For this review, take the finished solid that the model builds, in its own axes (mm). A direction names the side the tool comes from. Coordinates: 2 decimals unless noted, no trailing zeros. Write each loop counter-clockwise with the first axis right and the second up, starting at its lowest first coordinate (ties: lowest second). Pieces come first, ordered by that corner, then holes.
```python
from build123d import *

# Parameters (mm, degrees)
SKETCH_1_R               = 30
EXTRUDE_1_DEPTH          = 3
SKETCH_2_W               = 11
SKETCH_2_H               = 11
EXTRUDE_2_DEPTH          = 4
SKETCH_4_R               = 6
CUT_EXTRUDE_1_DEPTH      = 25
SKETCH_5_R               = 9
CUT_EXTRUDE_2_DEPTH      = 9
CUT_EXTRUDE_START        = 7.85
SKETCH_6_R               = 10
SKETCH_6_R_2             = 9
CUT_EXTRUDE_3_DEPTH      = 1.1
SKETCH_8_R               = 26.5
EXTRUDE_3_DEPTH          = 5
CUT_EXTRUDE_4_DEPTH      = 92.299851037
CUT_EXTRUDE_4_DEPTH_BACK = 92.299851037
SKETCH_7_R               = 15
SKETCH_10_R              = 2.25
CUT_EXTRUDE_5_DEPTH      = 17


with BuildPart() as part:
    # Sketch 1 → Extrude 1 (new body)
    with BuildSketch(Plane.XY):
        Circle(SKETCH_1_R)
    extrude(amount=EXTRUDE_1_DEPTH)



with BuildPart() as body_2:
    # Sketch 2 → Revolve 1 (revolve)
    with BuildSketch(Plane.XY.offset(3)):
        with Locations((68.415621645, -0.125)):
            Rectangle(SKETCH_2_W, SKETCH_2_H)
    revolve(axis=Axis((73.915621645, 22.717290725, 3), (0, -1, 0)))


with BuildPart() as part_1:
    add(part.part)

    add(body_2.part)  # Extrude 2 merges body 2
    # Sketch 3 → Extrude 2 (add, symmetric)
    with BuildSketch(Plane.XY.offset(3)):
        with BuildLine():
            Line((11.214731114, 27.824985284), (66.915621645, 5.375))
            Line((66.915621645, 5.375), (66.915621645, -4))
            Line((66.915621645, -4), (11.80104521, -27.581430926))
            ThreePointArc((11.80104521, -27.581430926), (-29.998320441, -0.317444067), (11.214731114, 27.824985284))
        make_face()
    extrude(amount=EXTRUDE_2_DEPTH, both=True)

    # Sketch 4 → Cut-Extrude 1 (cut)
    with BuildSketch(Plane.XZ.offset(5.625)):
        with Locations(Location((73.915621645, 3, 0), (0, 0, 270))):
            Circle(SKETCH_4_R)
    extrude(amount=-CUT_EXTRUDE_1_DEPTH, mode=Mode.SUBTRACT)

    # Sketch 5 → Cut-Extrude 2 (cut)
    with BuildSketch(Plane.XZ.offset(5.625)):
        with Locations(Location((73.915621645, 3, 0), (0, 0, 270))):
            Circle(SKETCH_5_R)
    extrude(amount=-CUT_EXTRUDE_2_DEPTH, mode=Mode.SUBTRACT)

    # Sketch 6 → Cut-Extrude 3 (cut)
    # profile 1 of 2: a face of its own
    with BuildSketch(Plane.XZ.offset(-3.375).offset(CUT_EXTRUDE_START)):
        with Locations(Location((73.915621645, 3, 0), (0, 0, 270))):
            Circle(SKETCH_6_R)
        with Locations(Location((73.915621645, 3, 0), (0, 0, 270))):
            Circle(SKETCH_6_R_2, mode=Mode.SUBTRACT)
    # profile 2 of 2: a face of its own
    with BuildSketch(Plane.XZ.offset(-3.375).offset(CUT_EXTRUDE_START)):
        with Locations(Location((73.915621645, 3, 0), (0, 0, 270))):
            Circle(SKETCH_6_R_2)
    extrude(amount=-CUT_EXTRUDE_3_DEPTH, mode=Mode.SUBTRACT)

    # Sketch 8 → Extrude 3 (add, symmetric)
    with BuildSketch(Plane(origin=(0, 0, 3), x_dir=(-1, 0, 0), z_dir=(0, 0, -1))):
        with Locations(Location((0, 0, 0), (0, 0, 180))):
            Circle(SKETCH_8_R)
    extrude(amount=EXTRUDE_3_DEPTH, both=True)

    # Sketch 7 → Cut-Extrude 4 (cut, two sides: drawn at the far end of the back side and taken through both)
    with BuildSketch(Plane.XY.offset(7).offset(-CUT_EXTRUDE_4_DEPTH_BACK)):
        with Locations(Location((0, 0, 0), (0, 0, 180))):
            Circle(SKETCH_7_R)
        with BuildLine():
            Line((25.989694724, -14.984517615), (51.662735414, -4))
            Line((51.662735414, -4), (29.732137495, -4))
            ThreePointArc((29.732137495, -4), (28.397104663, -9.674939108), (25.989694724, -14.984517615))
        make_face()
        with BuildLine():
            Line((29.732137495, 4), (51.662735414, 4))
            Line((51.662735414, 4), (25.989694724, 14.984517615))
            ThreePointArc((25.989694724, 14.984517615), (28.397104663, 9.674939108), (29.732137495, 4))
        make_face()
    extrude(amount=CUT_EXTRUDE_4_DEPTH + CUT_EXTRUDE_4_DEPTH_BACK, mode=Mode.SUBTRACT)

    # Sketch 10 → Cut-Extrude 5 (cut)
    with BuildSketch(Plane.XY.offset(8)):
        with Locations((21.75, 0)):
            Circle(SKETCH_10_R)
        with Locations((13.980630511, -16.661466638)):
            Circle(SKETCH_10_R)
        with Locations(Location((-21.75, 0, 0), (0, 0, 180))):
            Circle(SKETCH_10_R)
        with Locations(Location((-13.980630511, -16.661466638, 0), (0, 0, 180))):
            Circle(SKETCH_10_R)
        with Locations(Location((13.980630511, 16.661466638, 0), (0, 0, 180))):
            Circle(SKETCH_10_R)
        with Locations((-13.980630511, 16.661466638)):
            Circle(SKETCH_10_R)
    extrude(amount=-CUT_EXTRUDE_5_DEPTH, mode=Mode.SUBTRACT)


solid = part_1.part
```
1) Consider section D-D (z = 3.25). Count the separate pieces of the cut face and the enclosed holes in it, then the cut area to 3 significant figures.
2) Consider section C-C (x = 28). Give the boundary of the cut face in (y, z), then the cut area to 3 significant figures.
3) Clearance check with flat-ended pins moving along their axes: P1, Ø6.5, axis at x = 77, z = -0.5, coming from the -Y side (3 decimals); P2, Ø10, axis at x = -15, y = 14.5, coming from the +Z side; P3, Ø6.5, axis at x = 43.5, z = 3, coming from the +Y side. State where each tip first meets the part, or that it passes through.
4) For L1, parallel to X at y = -5.3, z = 3; L2, parallel to X at y = -6, z = 4.5; L3, parallel to X at y = -5.05, z = 3, list the stretches that pass through material, from the lowest coordinate up.
5) Consider section B-B (x = 76). Give the boundary of the cut face in (y, z) (3 decimals).
6) Consider section A-A (y = 7). Give the boundary of the cut face in (x, z).
7) The part is to be moulded in two halves that separate along Y. For faces 5 (the face through (-3.45, -26.274, 7.493)), 6 (the face through (72, -3.375, 12)), 7 (the face through (68, 4, 4)), say which applies: pulls with the +Y half, pulls with the -Y half, needs draft (parallel to the pull), parting line crosses it, or undercut.
8) Tool access review of faces 1 (the face through (-3.45, -26.274, -1.507)), 2 (the face through (65.13, -0.05, 4.95)), 3 (the face through (39.006, 9.415, 2.944)), 4 (the face through (72, -4.475, 12)): name each direction out of +Z, -Z, +X, -X, +Y, -Y from which nothing blocks a thin tool from reaching the whole face with its end or side.
Results:
1. separate pieces: 2
1. enclosed holes: 9
1. area: 2,860 mm2
2. outline: (-20.65, -1) - (-14.12, -1) - (-14.12, 7) - (-20.65, 7) - close; (-10.77, -1) - (10.77, -1) - (10.77, 7) - (-10.77, 7) - close; (14.12, -1) - (21.06, -1) - (21.06, 7) - (14.12, 7) - close
2. area: 280 mm2
3. P1: stops at y = 3.375
3. P2: stops at z = 8
3. P3: stops at y = 16.12
4. L1: x = -29.53 to -14.03, 14.03 to 29.53, 48.62 to 64.92, 82.92 to 84.92
4. L2: x = -29.39 to -13.75, 13.75 to 29.39, 46.99 to 62.24
4. L3: x = -29.57 to -14.12, 14.12 to 29.57, 49.21 to 64.92, 82.92 to 84.92
5. outline: (-5.625, -7.801) - (5.375, -7.801) - (5.375, -2.626) - (3.375, -2.626) - (3.375, -5.755) - (-3.375, -5.755) - (-3.375, -6.78) - (-4.475, -6.78) - (-4.475, -5.755) - (-5.625, -5.755) - close; (-5.625, 11.755) - (-4.475, 11.755) - (-4.475, 12.78) - (-3.375, 12.78) - (-3.375, 11.755) - (3.375, 11.755) - (3.375, 8.626) - (5.375, 8.626) - (5.375, 13.801) - (-5.625, 13.801) - close
6. outline: (-29.17, -1) - (-25.56, -1) - (-25.56, -2) - (-13.27, -2) - (-13.27, 8) - (-25.56, 8) - (-25.56, 7) - (-29.17, 7) - close; (13.27, -2) - (25.56, -2) - (25.56, -1) - (29.17, -1) - (29.17, 7) - (25.56, 7) - (25.56, 8) - (13.27, 8) - close; (44.65, -1) - (62.88, -1) - (62.88, 7) - (44.65, 7) - close
7. face 5: parting line crosses it
7. face 6: undercut
7. face 7: needs draft
8. face 1: -Z
8. face 2: -Y
8. face 3: +Z, -Z
8. face 4: none
